Design review of the part built by this model. Coordinates are the model's own, in mm. A direction names the side the tool comes from. Coordinates: 2 decimals unless noted, no trailing zeros. Loops run counter-clockwise (first coordinate to the right, second up) from the corner with the lowest first, then second, coordinate; pieces in that order, holes last. Notation, with made-up numbers: (9.25, 34.5) -> (49.25, 34.5) arc R15 cw to (49.25, 62.5) -> close; hole circle Ø6 at (41, 64.5). An arc over 180 degrees is marked (long way). Answer in a Markdown table with one row per item.
Autodesk Inventor part; units mm, degrees
ref_plane "YZ Plane" through (0, 0, 0) normal (1, 0, 0) x (0, 1, 0)
ref_plane "XZ Plane" through (0, 0, 0) normal (0, 1, 0) x (-1, 0, 0)
ref_plane "XY Plane" through (0, 0, 0) normal (0, 0, 1) x (1, 0, 0)
sketch "Sketch1" plane through (0, 0, 0) normal (0, 0, 1) x (1, 0, 0)
  line L0 (-58, 40) -> (58, 40)
  line L1 (70, 28) -> (70, -28)
  line L2 (58, -40) -> (-58, -40)
  line L3 (-70, -28) -> (-70, 28)
  arc A0 (70, 28) -> (58, 40) centre (58, 28) ccw
  arc A1 (58, -40) -> (70, -28) centre (58, -28) ccw
  line L4 (-58, 40) -> (-70, 28)
  line L5 (-70, -28) -> (-58, -40)
  line L6 (-70, 0) -> (70, 0) construction
  circle A2 centre (-60, 30) radius 2.6
  circle A3 centre (60, 30) radius 2.6
  line L7 (66.4853, 36.4853) -> (58, 28) construction
  circle A4 centre (-60, -30) radius 2.6
  circle A5 centre (60, -30) radius 2.6
  point P0 (0, 0)
  point P1 (-70, 40)
  point P2 (-70, -40)
  point P3 (0, 40)
  dimension "d0" = 140
  dimension "d1" = 80
  dimension "d2" = 12
  dimension "d3" = 12
  dimension "d4" = 12
  dimension "d5" = 12
  dimension "d6" = 12
  dimension "d7" = 5.2
  dimension "d8" = 120
  dimension "d9" = 60
extrude "Extrusion1" add sketch "Sketch1" along normal mid plane 12
sketch "Sketch2" plane through (-70, -28, 6) normal (-1, 0, 0) x (0, 0, 1)
  line L0 (-12, 68) -> (0, 68)
  point P0 (-6, 28)
  point P1 (-6, 33)
  dimension "d12" = 35
hole "Hole1" at (-70, 5, 0) direction (1, 0, 0) diameter 6 depth 88 tip angle 118
sketch "Sketch3" plane through (0, 0, 6) normal (0, 0, 1) x (1, 0, 0)
  line L0 (70, -28) -> (70, 28)
  line L1 (-70, 28) -> (-70, -28)
  circle A0 centre (22, 4) radius 25 construction
  line L2 (-70, 2) -> (-70, 8)
  line L3 (-70, 2) -> (-70, 8)
  line L4 (18, 8) -> (18, 2)
  line L5 (18, 5) -> (-70, 5) construction
  circle A1 centre (-35, 5) radius 5.5
  circle A2 centre (-35, 25) radius 5.5
  circle A3 centre (-35, 25) radius 3.25
  circle A4 centre (-35, -15) radius 5.5
  circle A5 centre (-35, -15) radius 3.25
  circle A6 centre (-35, 15) radius 2.5
  circle A7 centre (-35, -5) radius 2.5
  circle A8 centre (-35, 5) radius 3
  line L6 (58, 40) -> (-58, 40)
  point P0 (0, 0)
  point P1 (22, 29)
  point P2 (-3, 4)
  point P3 (22, -21)
  point P4 (47, 4)
  dimension "d22" = 50
  dimension "d20" = 48
  dimension "d25" = 360
  dimension "d27" = 11
  dimension "d28" = 35
  dimension "d30" = 11
  dimension "d31" = 6.5
  dimension "d32" = 20
  dimension "d33" = 5
  dimension "d34" = 10
  dimension "d51" = 6
  dimension "d59" = 36
hole "Hole2" at (22, 29, 6) at (47, 4, 6) at (22, -21, 6) at (-3, 4, 6) direction (0, 0, -1) diameter 4.134 depth 12
extrude "Extrusion2" cut sketch "Sketch3" against normal through all contours A3 | A5 | A6 | A7
extrude "Extrusion3" cut sketch "Sketch3" along normal blind 6 from surface at -12 contours A2 | A4
extrude "Extrusion4" cut sketch "Sketch3" against normal blind 1.5 contours A1 | A8
extrude "Extrusion5" cut sketch "Sketch3" against normal up to surface contours A8
sketch "Sketch4" plane through (-70, -28, 6) normal (-1, 0, 0) x (0, 0, 1)
  circle A0 centre (-6, 33) radius 3
  point P0 (-6, 28)
hole "Hole3" at (-70, 5, 0) direction (1, 0, 0) diameter 6.647 depth 15
properties part number "Base"
(1) Take a section at A-A on x = -60. Give the boundary of the cut face in (y, z).
Evaluation:
| item | result |
|---|---|
| outline | (-38, -6) -> (-32.6, -6) -> (-32.6, 6) -> (-38, 6) -> close; (-27.4, -6) -> (27.4, -6) -> (27.4, 6) -> (-27.4, 6) -> close; (32.6, -6) -> (38, -6) -> (38, 6) -> (32.6, 6) -> close; hole circle Ø6.65 at (5, 0) |
(2) Take a section at C-C on x = -7.5. Give the boundary of the cut face in (y, z), and give its area (3 significant figures).
Evaluation:
| item | result |
|---|---|
| outline | (-40, -6) -> (40, -6) -> (40, 6) -> (-40, 6) -> close; hole circle Ø6 at (5, 0) |
| area | 932 mm² |
(3) Take a section at D-D on x = -35. Count the separate pieces of the cut face and the enclosed holes in it, and give its area (3 significant figures).
Evaluation:
| item | result |
|---|---|
| separate pieces | 5 |
| enclosed holes | 0 |
| area | 572 mm² |
(4) Draft analysis for pull direction X (two halves, no side actions). For faces 4 (the flat face through (-70, 0, 0)), 5 (the cylindrical face through (21.38, -22.97, -0.08)), 6 (the flat face through (1, -40, 0)), state which applies: pulls with the +X half, pulls with the -X half, needs draft (parallel to the pull), parting line crosses it, or undercut.
Evaluation:
| item | result |
|---|---|
| face 4 | pulls with the -X half |
| face 5 | undercut |
| face 6 | needs draft |
(5) For pin 1 (6.5 mm diameter, centred on x = -35, y = 5, fed in from +Z); pin 2 (5.5 mm diameter, centred on y = 5, z = 0, fed in from -X); pin 3 (3.5 mm diameter, centred on x = -37.5, y = -17, fed in from -Z), all flat-tipped, find the tip position at first contact; note any pin that passes through.
Evaluation:
| item | result |
|---|---|
| pin 1 | stops at z = 4.5 |
| pin 2 | stops at x = 18.15 |
| pin 3 | stops at z = 0 |
(6) Take a section at B-B on x = 47. Give the boundary of the cut face in (y, z).
Evaluation:
| item | result |
|---|---|
| outline | (-40, -6) -> (1.93, -6) -> (1.93, 6) -> (-40, 6) -> close; (6.07, -6) -> (40, -6) -> (40, 6) -> (6.07, 6) -> close |
(7) Tool access review of faces 1 (the cylindrical face through (-18, 6.8, -2.4)), 2 (the cylindrical face through (-39.4, -11.7, -3)), 3 (the cylindrical face through (-35, 8, 3)): name each direction out of +Z, -Z, +X, -X, +Y, -Y from which nothing blocks a thin tool from reaching the whole face with its end or side.
Evaluation:
| item | result |
|---|---|
| face 1 | -X |
| face 2 | -Z |
| face 3 | +Z |
(8) To check wall thickness, follow probe 1 along Y at (x, z) = (-35, -4.05); probe 2 along Y at (x, z) = (22, -1); probe 3 along Y at (x, z) = (-35, 4.95). State the ranges of each line that lie inside material, in increasing order.
Evaluation:
| item | result |
|---|---|
| probe 1 | y = -40 to -20.5, -9.5 to -7.5, -2.5 to 12.5, 17.5 to 19.5, 30.5 to 40 |
| probe 2 | y = -40 to -23.07, -18.93 to 26.93, 31.07 to 40 |
| probe 3 | y = -40 to -18.25, -11.75 to -7.5, -2.5 to -0.5, 10.5 to 12.5, 17.5 to 21.75, 28.25 to 40 |
